Geometry check sheet. Reference: the model listing, model coordinates, mm. A direction names the side the tool comes from. Give positions to 0.01 mm unless a question says otherwise; leave off trailing zeros. Order: outer loops, then holes, each group sorted by start corner. A loop starts at its lowest first (then second) coordinate and runs counter-clockwise, first axis right, second up.
```python
from build123d import *

# Parameters (mm, degrees)
SALIENTE_EXTRUIR1_DEPTH                              = 10.8
CORTAR_EXTRUIR1_DEPTH                                = 2.2
SALIENTE_EXTRUIR2_DEPTH                              = 2.2
SALIENTE_EXTRUIR3_DEPTH                              = 2.2
CROQUIS5_W                                           = 16
CROQUIS5_H                                           = 2.4
SALIENTE_EXTRUIR4_DEPTH                              = 4.4
CROQUIS6_W                                           = 16
CROQUIS6_H                                           = 6.2
CORTAR_EXTRUIR2_DEPTH                                = 21
REFRENTADO_PARA_PERNO_CON_CABEZA_HEXAGON_D           = 8.45
REFRENTADO_PARA_PERNO_CON_CABEZA_HEXAGON_CBORE_D     = 15
REFRENTADO_PARA_PERNO_CON_CABEZA_HEXAGON_CBORE_DEPTH = 7.3
REFRENTADO_PARA_TORNILLO_CON_CABEZA_HEXA_D           = 3
REFRENTADO_PARA_TORNILLO_CON_CABEZA_HEXA_DEPTH       = 10.8
REFRENTADO_PARA_TORNILLO_CON_CABEZA_HEXA_CBORE_D     = 6.2
REFRENTADO_PARA_TORNILLO_CON_CABEZA_HEXA_CBORE_DEPTH = 3
REDONDEO1_R                                          = 1
CHAFL_N1_SIZE                                        = 0.25
REDONDEO2_R                                          = 0.5


with BuildPart() as part:
    # Croquis1 → Saliente-Extruir1 (new body)
    with BuildSketch(Plane(origin=(0, 0, 0), x_dir=(1, 0, 0), z_dir=(0, 1, 0))):
        Polygon((21, -17), (21, 17), (17, 21), (-17, 21), (-21, 17), (-21, -17), (-17, -21), (17, -21), align=None)
    extrude(amount=-SALIENTE_EXTRUIR1_DEPTH)

    # Croquis2 → Cortar-Extruir1 (cut)
    with BuildSketch(Plane.XZ.offset(10.8)):
        Polygon((-21, 17), (-21, -14.100780618), (-14.100780618, -21), (14.100780618, -21), (21, -14.100780618), (21, 17), (17, 21), (-17, 21), align=None)
    extrude(amount=-CORTAR_EXTRUIR1_DEPTH, mode=Mode.SUBTRACT)

    # Croquis3 → Saliente-Extruir2 (add)
    with BuildSketch(Plane.XZ.offset(8.6)):
        Polygon((-21, 17), (-17, 21), (-14.100780618, 21), (-21, 14.100780618), align=None)
    extrude(amount=SALIENTE_EXTRUIR2_DEPTH)

    # Croquis4 → Saliente-Extruir3 (add)
    with BuildSketch(Plane.XZ.offset(8.6)):
        Polygon((21, 17), (21, 14.100780618), (14.100780618, 21), (17, 21), align=None)
    extrude(amount=SALIENTE_EXTRUIR3_DEPTH)

    # Croquis5 → Saliente-Extruir4 (add)
    with BuildSketch(Plane(origin=(21, 0, 0), x_dir=(0, 0, -1), z_dir=(1, 0, 0))):
        with Locations((0, -1.2)):
            Rectangle(CROQUIS5_W, CROQUIS5_H)
    extrude(amount=SALIENTE_EXTRUIR4_DEPTH)

    # Croquis6 → Cortar-Extruir2 (cut)
    with BuildSketch(Plane(origin=(21, 0, 0), x_dir=(0, 0, -1), z_dir=(1, 0, 0))):
        with Locations((0, -5.5)):
            Rectangle(CROQUIS6_W, CROQUIS6_H)
    extrude(amount=-CORTAR_EXTRUIR2_DEPTH, mode=Mode.SUBTRACT)

    # Refrentado para perno con cabeza hexagonal de M81 (through all)
    with Locations(Plane(origin=(0, -8.6, 0), x_dir=(-1, 0, 0), z_dir=(0, -1, 0))):
        with Locations((0, 0)):
            CounterBoreHole(REFRENTADO_PARA_PERNO_CON_CABEZA_HEXAGON_D / 2, REFRENTADO_PARA_PERNO_CON_CABEZA_HEXAGON_CBORE_D / 2, REFRENTADO_PARA_PERNO_CON_CABEZA_HEXAGON_CBORE_DEPTH)

    # Refrentado para tornillo con cabeza hexagonal de M2.51
    with Locations(Plane(origin=(0, 0, 0), x_dir=(1, 0, 0), z_dir=(0, 1, 0))):
        with Locations((15.5, -15.5), (-15.5, -15.5), (-15.5, 15.5), (15.5, 15.5)):
            CounterBoreHole(REFRENTADO_PARA_TORNILLO_CON_CABEZA_HEXA_D / 2, REFRENTADO_PARA_TORNILLO_CON_CABEZA_HEXA_CBORE_D / 2, REFRENTADO_PARA_TORNILLO_CON_CABEZA_HEXA_CBORE_DEPTH, depth=REFRENTADO_PARA_TORNILLO_CON_CABEZA_HEXA_DEPTH)

    # Redondeo1
    redondeo1_edges = [part.edges().sort_by_distance(p)[0] for p in [
        (-21, -5.4, -17),
        (-17, -5.4, -21),
        (17, -5.4, -21),
        (21, -5.4, -17),
        (21, -5.4, 17),
        (-21, -5.4, 17),
        (-17, -5.4, 21),
        (17, -5.4, 21),
        (25.4, -1.2, -8),
        (25.4, -1.2, 8),
    ]]
    fillet(redondeo1_edges, radius=REDONDEO1_R)

    # Chaflán1
    chafl_n1_edges = [part.edges().sort_by_distance(p)[0] for p in [
        (-4.225, 0, 0),
        (-18.6, 0, -15.5),
        (-18.6, 0, 15.5),
        (12.4, 0, 15.5),
    ]]
    chamfer(chafl_n1_edges, length=CHAFL_N1_SIZE)

    # Redondeo2
    redondeo2_edges = [part.edges().sort_by_distance(p)[0] for p in [
        (25.4, 0, 0),
        (19, 0, 19),
        (21, 0, 12.292893219),
        (22.7, 0, 8),
        (22.7, 0, -8),
        (19, 0, -19),
        (0, 0, -21),
        (-19, 0, -19),
        (-21, 0, 0),
        (-19, 0, 19),
        (0, 0, 21),
        (20.923879533, 0, 16.96846987),
        (20.923879533, 0, -16.96846987),
        (-20.923879533, 0, -16.96846987),
        (16.96846987, 0, 20.923879533),
        (16.96846987, 0, -20.923879533),
        (-16.96846987, 0, 20.923879533),
        (-16.96846987, 0, -20.923879533),
        (25.107106781, 0, 7.707106781),
        (-20.923879533, 0, 16.96846987),
        (25.107106781, 0, -7.707106781),
        (21, 0, -12.292893219),
    ]]
    fillet(redondeo2_edges, radius=REDONDEO2_R)


solid = part.part
```
Q1. Cross-section at D-D, the plane z = 0. Record the boundary of the cut face in (x, y) (3 decimals), and give its area (3 significant figures).
Q2. Thickness scan on L1, parallel to X at y = -2.1, z = -15.5; L2, parallel to Z at x = 15.5, y = -7; L3, parallel to Z at x = -15.5, y = -7.4. Record the ranges inside material, lowest first.
Q3. Access from +Z, -Z, +X, -X, +Y, -Y to the whole of each face (thin tool, end or side, straight path). Record for faces 1 (the face through (11, -6, -8)), 2 (the face through (-7.154, -5.001, -2.253)), 3 (the face through (-14.07, -1.61, -12.75)).
Q4. Gauge pin test, flat ends, axial feed: P1, Ø5, axis at y = -4.5, z = 15, coming from the +X side; P2, Ø5, axis at x = 15.5, z = 15.5, coming from the +Y side; P3, Ø3.5, axis at x = 15.5, z = -15.5, coming from the -Y side. Record the tip position at first contact, or that the pin passes through.
Q5. Cross-section at C-C, the plane y = -7.5. Record the boundary of the cut face in (x, z).
Q6. Cross-section at A-A, the plane z = 15.5. Give the number of separate pieces and of enclosed holes in the cut face, and give its area (3 significant figures).
Q7. Release check for a two-part mould opening along Z. For faces 4 (the face through (-18.918, -0.143, -18.87)), 5 (the face through (-17.5, -9.7, 17.6)), 6 (the face through (-19, -6, 19)) record: pulls with the +Z half, pulls with the -Z half, needs draft (parallel to the pull), parting line crosses it, or undercut.
Answers follow:
1. outline: (-21, -8.6) - (-7.5, -8.6) - (-7.5, -1.3) - (-4.225, -1.3) - (-4.225, -0.25) - (-4.475, 0) - (-20.5, 0) arc R0.5 ccw to (-21, -0.5) - close; (4.225, -1.3) - (7.5, -1.3) - (7.5, -2.4) - (25.4, -2.4) - (25.4, -0.5) arc R0.5 ccw to (24.9, 0) - (4.475, 0) - (4.225, -0.25) - close
1. area: 167 mm2
2. L1: x = -21 to -18.6, -12.4 to 12.4, 18.6 to 21
2. L2: z = -21 to -17, -14 to -8, 8 to 14, 17 to 21
2. L3: z = -21 to -17, -14 to 14, 17 to 21
3. face 1: +X, -Y
3. face 2: -Y
3. face 3: +Y
4. P1: stops at x = 21
4. P2: stops at y = -3
4. P3: stops at y = -8.6
5. outline: (-21, -16.59) arc R1 ccw to (-20.71, -17.29) - (-17.29, -20.71) arc R1 ccw to (-16.59, -21) - (16.59, -21) arc R1 ccw to (17.29, -20.71) - (20.71, -17.29) arc R1 ccw to (21, -16.59) - (21, -8) - (0, -8) - (0, -7.5) arc R7.5 cw to (0, 7.5) - (0, 8) - (21, 8) - (21, 16.59) arc R1 ccw to (20.71, 17.29) - (17.29, 20.71) arc R1 ccw to (16.59, 21) - (-16.59, 21) arc R1 ccw to (-17.29, 20.71) - (-20.71, 17.29) arc R1 ccw to (-21, 16.59) - close; hole circle Ø3 at (-15.5, -15.5); hole circle Ø3 at (-15.5, 15.5); hole circle Ø3 at (15.5, -15.5); hole circle Ø3 at (15.5, 15.5)
6. separate pieces: 3
6. enclosed holes: 0
6. area: 296 mm2
7. face 4: pulls with the -Z half
7. face 5: undercut
7. face 6: pulls with the +Z half
